from build123d import *

# Parameters (mm, degrees)
SKETCH1_R           = 6.650000000000002
BOSS_EXTRUDE1_DEPTH = 6
BOSS_EXTRUDE2_DEPTH = 32
FILLET1_R           = 4
CHAMFER1_SIZE       = 4
CHAMFER2_SIZE       = 1
SKETCH3_R           = 8.699999999995331
CUT_EXTRUDE1_DEPTH  = 1.5


with BuildPart() as part:
    # Sketch1 → Boss-Extrude1 (new body)
    with BuildSketch(Plane.XY):
        Polygon((15.23657634098733, 19.422325849528544), (24.56734683192624, 2.4136009694730585), (24.12897763398666, 2.173117193933393), (-14.79820714304776, -19.1818420739889), (-15.236576340987371, -19.42232584952858), (-24.567346831926308, -2.4136009694729568), (-24.12897763398673, -2.173117193933293), (14.798207143047753, 19.181842073988882), align=None)
        Circle(SKETCH1_R, mode=Mode.SUBTRACT)
    extrude(amount=-BOSS_EXTRUDE1_DEPTH)

    # Sketch2 → Boss-Extrude2 (add)
    with BuildSketch(Plane.XY):
        Polygon((24.56734683192624, 2.4136009694730585), (15.23657634098733, 19.422325849528544), (18.743529924503946, 21.34619605384586), (28.07430041544286, 4.337471173790374), align=None)
        Polygon((-24.567346831926308, -2.4136009694729568), (-15.236576340987371, -19.42232584952858), (-18.743529924503996, -21.346196053845887), (-28.074300415442934, -4.337471173790264), align=None)
    extrude(amount=-BOSS_EXTRUDE2_DEPTH)

    # Fillet1
    fillet1_edges = [part.edges().sort_by_distance(p)[0] for p in [
        (19.901961586456785, 10.917963409500802, -6),
        (-19.90196158645684, -10.917963409500768, -6),
    ]]
    fillet(fillet1_edges, radius=FILLET1_R)

    # Chamfer1
    chamfer1_edges = [part.edges().sort_by_distance(p)[0] for p in [
        (23.408915169973405, 12.841833613818116, 0),
        (-23.408915169973465, -12.841833613818075, 0),
    ]]
    chamfer(chamfer1_edges, length=CHAMFER1_SIZE)

    # Chamfer2
    chamfer2_edges = [part.edges().sort_by_distance(p)[0] for p in [
        (26.32082362368455, 3.375536071631716, -32),
        (28.07430041544286, 4.337471173790374, -18),
        (24.56734683192624, 2.4136009694730585, -21),
        (19.901961586456785, 10.917963409500802, -32),
        (16.990053132745636, 20.384260951687203, -32),
        (15.23657634098733, 19.422325849528544, -21),
        (23.408915169973405, 12.841833613818116, -32),
        (18.743529924503946, 21.34619605384586, -18),
        (-26.32082362368462, -3.3755360716316103, -32),
        (-28.074300415442934, -4.337471173790264, -18),
        (-24.567346831926308, -2.4136009694729568, -21),
        (-19.90196158645684, -10.917963409500768, -32),
        (-16.990053132745683, -20.38426095168723, -32),
        (-15.236576340987371, -19.42232584952858, -21),
        (-23.408915169973465, -12.841833613818075, -32),
        (-18.743529924503996, -21.346196053845887, -18),
        (4.665385245469443, -8.504362440027757, -6),
        (-4.665385245469494, 8.504362440027792, -6),
        (-14.209413417681859, -18.858837312806703, -7.171572875253809),
        (-23.540183908620747, -1.8501124327511644, -7.171572875253809),
        (14.209413417681818, 18.85883731280668, -7.171572875253809),
        (23.54018390862069, 1.8501124327512626, -7.171572875253809),
        (-4.665385245469494, 8.504362440027798, 0),
        (4.66538524546943, -8.504362440027759, 0),
        (26.32082362368455, 3.375536071631717, -2.0000000000000004),
        (-16.99005313274572, -20.38426095168716, -2.0000000000000018),
        (16.990053132745686, 20.384260951687114, -1.9999999999999964),
        (-26.32082362368462, -3.3755360716316103, -2.000000000000001),
    ]]
    chamfer(chamfer2_edges, length=CHAMFER2_SIZE)

    # Sketch3 → Cut-Extrude1 (cut)
    with BuildSketch(Plane(origin=(0, 0, -6), x_dir=(-1, 0, 0), z_dir=(0, 0, -1))):
        Circle(SKETCH3_R)
    extrude(amount=-CUT_EXTRUDE1_DEPTH, mode=Mode.SUBTRACT)


solid = part.part
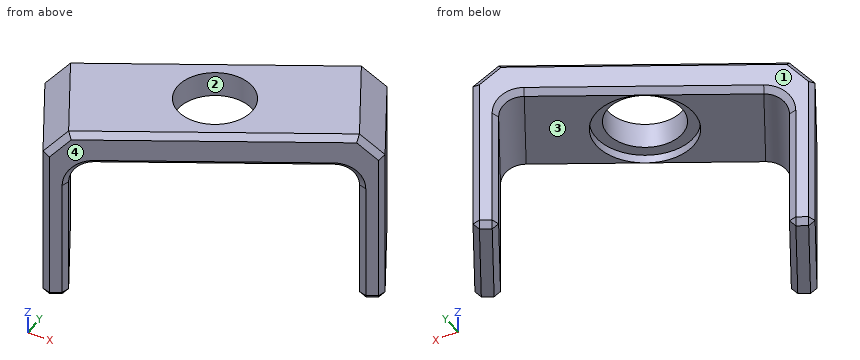
Work out the finished part from the listing and answer in its coordinate system (mm). Face numbers are marked on the shaded views. Round coordinates to 2 decimals unless told otherwise and drop trailing zeros. Write each loop counter-clockwise with the first axis right and the second up, starting at its lowest first coordinate (ties: lowest second). Pieces come first, ordered by that corner, then holes.
1) A cutting plane is placed at A-A (z = -18). Give the vertices of the cut face in (x, y), plus the area to 3 significant figures.
2) The mould has two halves that part along X. Classify the marked faces 1, 2, 3 and 4: pulls with the +X half, pulls with the -X half, needs draft (parallel to the pull), parting line crosses it, or undercut.
3) A cutting plane is placed at C-C (z = -3). Give the vertices of the cut face in (x, y), plus the area to 3 significant figures.
4) Straight lines are drawn through the part: line 1 (X direction, y = 0, z = -5.55); line 2 (X direction, y = 2.5, z = -2); line 3 (Y direction, x = 0, z = -4). For each, find the intervals that lie inside material, in ascending order.
5) A cutting plane is placed at B-B (x = 0). Give the vertices of the cut face in (y, z), plus the area to 3 significant figures.
6) Given pin 1 Ø15.5 at (x, y) = (0, 0) entering from -Z; pin 2 Ø2 at (y, z) = (16, -10.5) entering from +X (3 decimals); pin 3 Ø5 at (x, z) = (-22, -9.5) entering from +Y, each flat-ended and moving along its own axis, determine where each tip first touches the part or whether it passes through.
Completed:
1. outline: (-27.59, -5.21) - (-19.22, -20.47) - (-17.87, -20.87) - (-16.11, -19.9) - (-15.72, -18.55) - (-24.09, -3.29) - (-25.44, -2.89) - (-27.2, -3.86) - close; (15.72, 18.55) - (24.09, 3.29) - (25.44, 2.89) - (27.2, 3.86) - (27.59, 5.21) - (19.22, 20.47) - (17.87, 20.87) - (16.11, 19.9) - close
1. area: 151 mm2
2. face 1: pulls with the -X half
2. face 2: undercut
2. face 3: needs draft
2. face 4: pulls with the +X half
3. outline: (-26.72, -4.73) - (-18.35, -19.99) - (-16.63, -20.19) - (25.96, 3.18) - (26.72, 4.73) - (18.35, 19.99) - (16.63, 20.19) - (-25.96, -3.18) - close; hole circle Ø13.3 at (0, 0)
3. area: 855 mm2
4. line 1: x = -19.02 to -8.7, 8.7 to 19.02
4. line 2: x = -15.61 to -6.16, 6.16 to 24.72
4. line 3: y = -11.06 to -6.65, 6.65 to 11.06
5. outline: (-11.06, -5) - (-9.92, -6) - (-8.7, -6) - (-8.7, -4.5) - (-6.65, -4.5) - (-6.65, 0) - (-9.92, 0) - (-11.06, -1) - close; (6.65, -4.5) - (8.7, -4.5) - (8.7, -6) - (9.92, -6) - (11.06, -5) - (11.06, -1) - (9.92, 0) - (6.65, 0) - close
5. area: 44.5 mm2
6. pin 1: stops at z = -4.5
6. pin 2: stops at x = 22.225
6. pin 3: stops at y = -2.78
